from build123d import *

# Parameters (mm, degrees)
BOSS_EXTRU_1_DEPTH = 2.5
CHANFREIN1_SIZE    = 0.1


with BuildPart() as part:
    # Esquisse1 → Boss.-Extru.1 (new body)
    with BuildSketch(Plane.XY):
        Polygon((-114, 35), (114, 35), (114, -35), (-49.5, -35), (-49.5, -45), (-59.5, -45), (-59.5, -35), (-114, -35), align=None)
        with BuildLine():
            Line((-111.5, -27.5), (-111.5, 27.5))
            ThreePointArc((-111.5, 27.5), (-108, 31), (-104.5, 27.5))
            Line((-104.5, 27.5), (-104.5, -27.5))
            ThreePointArc((-104.5, -27.5), (-108, -31), (-111.5, -27.5))
        make_face(mode=Mode.SUBTRACT)
        with BuildLine():
            Line((-92.5, -27.5), (-92.5, 27.5))
            ThreePointArc((-92.5, 27.5), (-96, 31), (-99.5, 27.5))
            Line((-99.5, 27.5), (-99.5, -27.5))
            ThreePointArc((-99.5, -27.5), (-96, -31), (-92.5, -27.5))
        make_face(mode=Mode.SUBTRACT)
        with BuildLine():
            Line((-80.5, -27.5), (-80.5, 27.5))
            ThreePointArc((-80.5, 27.5), (-84, 31), (-87.5, 27.5))
            Line((-87.5, 27.5), (-87.5, -27.5))
            ThreePointArc((-87.5, -27.5), (-84, -31), (-80.5, -27.5))
        make_face(mode=Mode.SUBTRACT)
        with BuildLine():
            Line((-68.5, -27.5), (-68.5, 27.5))
            ThreePointArc((-68.5, 27.5), (-72, 31), (-75.5, 27.5))
            Line((-75.5, 27.5), (-75.5, -27.5))
            ThreePointArc((-75.5, -27.5), (-72, -31), (-68.5, -27.5))
        make_face(mode=Mode.SUBTRACT)
        with BuildLine():
            Line((-56.5, -27.5), (-56.5, 27.5))
            ThreePointArc((-56.5, 27.5), (-60, 31), (-63.5, 27.5))
            Line((-63.5, 27.5), (-63.5, -27.5))
            ThreePointArc((-63.5, -27.5), (-60, -31), (-56.5, -27.5))
        make_face(mode=Mode.SUBTRACT)
        with BuildLine():
            Line((-44.5, -27.5), (-44.5, 27.5))
            ThreePointArc((-44.5, 27.5), (-48, 31), (-51.5, 27.5))
            Line((-51.5, 27.5), (-51.5, -27.5))
            ThreePointArc((-51.5, -27.5), (-48, -31), (-44.5, -27.5))
        make_face(mode=Mode.SUBTRACT)
        with BuildLine():
            Line((-32.5, -27.5), (-32.5, 27.5))
            ThreePointArc((-32.5, 27.5), (-36, 31), (-39.5, 27.5))
            Line((-39.5, 27.5), (-39.5, -27.5))
            ThreePointArc((-39.5, -27.5), (-36, -31), (-32.5, -27.5))
        make_face(mode=Mode.SUBTRACT)
        with BuildLine():
            Line((-20.5, -27.5), (-20.5, 27.5))
            ThreePointArc((-20.5, 27.5), (-24, 31), (-27.5, 27.5))
            Line((-27.5, 27.5), (-27.5, -27.5))
            ThreePointArc((-27.5, -27.5), (-24, -31), (-20.5, -27.5))
        make_face(mode=Mode.SUBTRACT)
        with BuildLine():
            Line((-8.5, -27.5), (-8.5, 27.5))
            ThreePointArc((-8.5, 27.5), (-12, 31), (-15.5, 27.5))
            Line((-15.5, 27.5), (-15.5, -27.5))
            ThreePointArc((-15.5, -27.5), (-12, -31), (-8.5, -27.5))
        make_face(mode=Mode.SUBTRACT)
        with BuildLine():
            Line((3.5, -27.5), (3.5, 27.5))
            ThreePointArc((3.5, 27.5), (0, 31), (-3.5, 27.5))
            Line((-3.5, 27.5), (-3.5, -27.5))
            ThreePointArc((-3.5, -27.5), (0, -31), (3.5, -27.5))
        make_face(mode=Mode.SUBTRACT)
        with BuildLine():
            Line((15.5, -27.5), (15.5, 27.5))
            ThreePointArc((15.5, 27.5), (12, 31), (8.5, 27.5))
            Line((8.5, 27.5), (8.5, -27.5))
            ThreePointArc((8.5, -27.5), (12, -31), (15.5, -27.5))
        make_face(mode=Mode.SUBTRACT)
        with BuildLine():
            Line((27.5, -27.5), (27.5, 27.5))
            ThreePointArc((27.5, 27.5), (24, 31), (20.5, 27.5))
            Line((20.5, 27.5), (20.5, -27.5))
            ThreePointArc((20.5, -27.5), (24, -31), (27.5, -27.5))
        make_face(mode=Mode.SUBTRACT)
        with BuildLine():
            Line((39.5, -27.5), (39.5, 27.5))
            ThreePointArc((39.5, 27.5), (36, 31), (32.5, 27.5))
            Line((32.5, 27.5), (32.5, -27.5))
            ThreePointArc((32.5, -27.5), (36, -31), (39.5, -27.5))
        make_face(mode=Mode.SUBTRACT)
        with BuildLine():
            Line((51.5, -27.5), (51.5, 27.5))
            ThreePointArc((51.5, 27.5), (48, 31), (44.5, 27.5))
            Line((44.5, 27.5), (44.5, -27.5))
            ThreePointArc((44.5, -27.5), (48, -31), (51.5, -27.5))
        make_face(mode=Mode.SUBTRACT)
        with BuildLine():
            Line((63.5, -27.5), (63.5, 27.5))
            ThreePointArc((63.5, 27.5), (60, 31), (56.5, 27.5))
            Line((56.5, 27.5), (56.5, -27.5))
            ThreePointArc((56.5, -27.5), (60, -31), (63.5, -27.5))
        make_face(mode=Mode.SUBTRACT)
        with BuildLine():
            Line((75.5, -27.5), (75.5, 27.5))
            ThreePointArc((75.5, 27.5), (72, 31), (68.5, 27.5))
            Line((68.5, 27.5), (68.5, -27.5))
            ThreePointArc((68.5, -27.5), (72, -31), (75.5, -27.5))
        make_face(mode=Mode.SUBTRACT)
        with BuildLine():
            Line((87.5, -27.5), (87.5, 27.5))
            ThreePointArc((87.5, 27.5), (84, 31), (80.5, 27.5))
            Line((80.5, 27.5), (80.5, -27.5))
            ThreePointArc((80.5, -27.5), (84, -31), (87.5, -27.5))
        make_face(mode=Mode.SUBTRACT)
        with BuildLine():
            Line((99.5, -27.5), (99.5, 27.5))
            ThreePointArc((99.5, 27.5), (96, 31), (92.5, 27.5))
            Line((92.5, 27.5), (92.5, -27.5))
            ThreePointArc((92.5, -27.5), (96, -31), (99.5, -27.5))
        make_face(mode=Mode.SUBTRACT)
        with BuildLine():
            Line((111.5, -27.5), (111.5, 27.5))
            ThreePointArc((111.5, 27.5), (108, 31), (104.5, 27.5))
            Line((104.5, 27.5), (104.5, -27.5))
            ThreePointArc((104.5, -27.5), (108, -31), (111.5, -27.5))
        make_face(mode=Mode.SUBTRACT)
        Polygon((-51, -42.020725942), (-51, -37.979274058), (-54.5, -35.958548116), (-58, -37.979274058), (-58, -42.020725942), (-54.5, -44.041451884), align=None, mode=Mode.SUBTRACT)
    extrude(amount=BOSS_EXTRU_1_DEPTH)

    # Chanfrein1
    chanfrein1_edges = [part.edges().sort_by_distance(p)[0] for p in [
        (-52.75, -43.031088913, 2.5),
        (-51, -40, 2.5),
        (-52.75, -36.968911087, 2.5),
        (-56.25, -36.968911087, 2.5),
        (-58, -40, 2.5),
        (-56.25, -43.031088913, 2.5),
    ]]
    chamfer(chanfrein1_edges, length=CHANFREIN1_SIZE)


solid = part.part
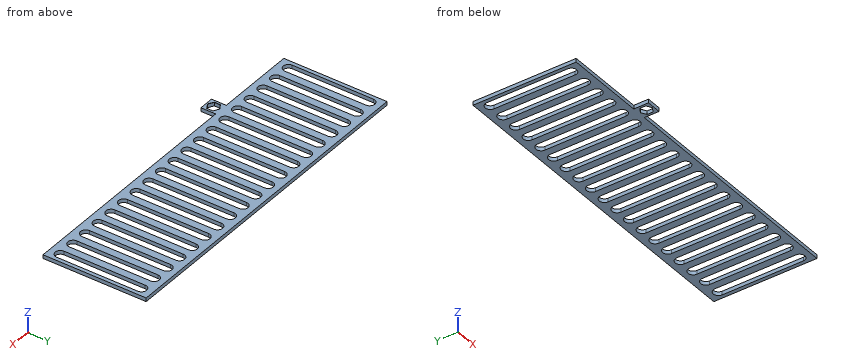
The listing builds one solid part. Answer for the finished solid, in the listing's coordinates (mm). Coordinates: 2 decimals unless noted, no trailing zeros. Loops run counter-clockwise (first coordinate to the right, second up) from the corner with the lowest first, then second, coordinate; pieces in that order, holes last. Notation, with made-up numbers: (42.25, 28.5) -> (46.25, 28.5) arc R20 cw to (46.25, 47.5) -> close; hole circle Ø6 at (59, 39). An arc over 180 degrees is marked (long way). Write item = value, one per line. Start each with the question number.
1) Straight lines are drawn through the part: line 1 (Y direction, x = -0.5, z = 1.55); line 2 (Y direction, x = -78.5, z = 2.35); line 3 (Y direction, x = 38, z = 1.4). For each, find the intervals that lie inside material, in ascending order. Write a range as from..to.
2) A cutting plane is placed at B-B (y = 25). Count the separate pieces of the cut face and the enclosed holes in it, then the cut area to 4 significant figures.
3) Given pin 1 Ø1.5 at (x, z) = (65.5, 0.5) entering from -Y, flat-ended and moving along its own axis, determine where the tip first touches the part or whether it passes through.
4) A cutting plane is placed at A-A (x = 48). Give the vertices of the cut face in (y, z).
Responses:
q1.line_1 = -35..-30.96, 30.96..35
q1.line_2 = -35..35
q1.line_3 = -35..-30.37, 30.37..35
q2.separate_pieces = 20
q2.enclosed_holes = 0
q2.area = 237.5 mm²
q3.pin_1 = -35
q4.outline = (-35, 0) -> (-31, 0) -> (-31, 2.5) -> (-35, 2.5) -> close; (31, 0) -> (35, 0) -> (35, 2.5) -> (31, 2.5) -> close
